The drawing under review shows one solid part. Ordinate dimensions are in mm from its lowest x, y, z. Coordinates: 2 decimals unless noted, no trailing zeros. Loops run counter-clockwise (first coordinate to the right, second up) from the corner with the lowest first, then second, coordinate; pieces in that order, holes last. Notation, with made-up numbers: M -33,33.25 L 15,33.25 A36 cw 15,71.25 Z; hole C 88,56.25 d4. An arc over 180 degrees is marked long. Put each result on its own line as item: value.
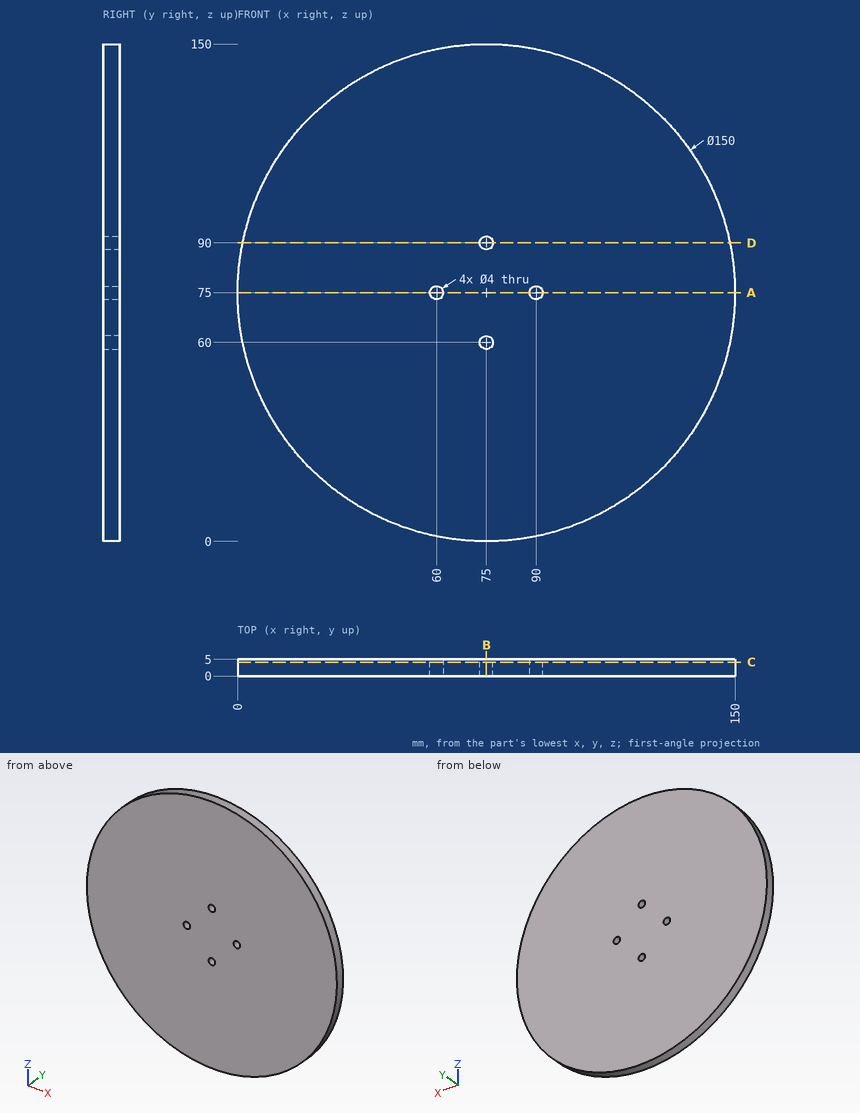
(1) Add section D-D (z = 90). Write out the cut boundary in (x, y), plus the area to 3 significant figures.
Determined:
outline: M 1.52,0 L 73,0 L 73,5 L 1.52,5 Z; M 77,0 L 148.48,0 L 148.48,5 L 77,5 Z
area: 715 mm^2
(2) Add section B-B (x = 75). Write out the cut boundary in (y, z).
Determined:
outline: M 0,0 L 5,0 L 5,58 L 0,58 Z; M 0,62 L 5,62 L 5,88 L 0,88 Z; M 0,92 L 5,92 L 5,150 L 0,150 Z
(3) Add section A-A (z = 75). Write out the cut boundary in (x, y), plus the area to 3 significant figures.
Determined:
outline: M 0,0 L 58,0 L 58,5 L 0,5 Z; M 62,0 L 88,0 L 88,5 L 62,5 Z; M 92,0 L 150,0 L 150,5 L 92,5 Z
area: 710 mm^2
(4) For pin 1 (3 mm diameter, centred on x = 25, y = 3.5, fed in from -Z); pin 2 (3 mm diameter, centred on x = 57, y = 4, fed in from +Z); pin 3 (3 mm diameter, centred on x = 75, z = 90, fed in from +Y); pin 4 (1 mm diameter, centred on x = 118, y = 4, fed in from +Z), all flat-tipped, find the tip position at first contact; note any pin that passes through.
Determined:
pin 1: stops at z = 17.79
pin 2: stops at z = 148.16
pin 3: passes through
pin 4: stops at z = 136.8
(5) Wall thickness on line 1 along Z through (x, y) = (90, 2.65); line 2 along Z through (x, y) = (22.5, 0.9); line 3 along X through (y, z) = (1.4, 134.5): over which ranges is each line inside the solid? List them lowest first. Write a range as [from, to].
Determined:
line 1: z = [1.52, 73], [77, 148.48]
line 2: z = [21.44, 128.56]
line 3: x = [29.34, 120.66]
(6) Add section C-C (y = 4.2). Write out the cut boundary in (x, z).
Determined:
outline: C 75,75 d150; hole C 60,75 d4; hole C 75,60 d4; hole C 75,90 d4; hole C 90,75 d4
